Geometry check sheet. Reference: the model listing, model coordinates, mm. Face numbers are marked on the shaded views. A direction names the side the tool comes from. Give positions to 0.01 mm unless a question says otherwise; leave off trailing zeros. Write each loop counter-clockwise with the first axis right and the second up, starting at its lowest first coordinate (ties: lowest second). Pieces come first, ordered by that corner, then holes. Notation, with made-up numbers: (62, -14.5) -> (105, -14.5) arc R16 ccw to (105, -8.5) -> close; hole circle Ø11 at (47.25, -4.75). An arc over 180 degrees is marked (long way). Write item = value, one per line. Start each with the question number.
1. Mould release check, pull along X, two halves, no side actions. Record for the marked faces 1, 2, 3 and 4: pulls with the +X half, pulls with the -X half, needs draft (parallel to the pull), parting line crosses it, or undercut.
2. Depth check by flat-ended pin: P1, Ø2.5, axis at x = 3.5, y = 17.5, coming from the -Z side; P2, Ø1.4, axis at x = -10, z = -10.5, coming from the -Y side; P3, Ø1.6, axis at y = 17, z = 4, coming from the -X side. Enter the tip coordinate at first touch or a pass-through.
3. Cross-section at D-D, the plane y = 17. Record the cut outline in (x, z), plus the area to 3 significant figures.
4. Thickness scan on line 1 along Z through (x, y) = (10.25, 8); line 2 along Z through (x, y) = (-10.75, 6.25); line 3 along X through (y, z) = (9.25, -9.75). Record the ranges inside material, lowest first.
5. Set-up check for the marked faces 5 and 6: record each of +Z, -Z, +X, -X, +Y, -Y from which the full face is reachable in a straight line by a thin tool's end or side.
6. Cross-section at A-A, the plane y = 3.5. Record the cut outline in (x, z).
```python
from build123d import *

# Parameters (mm, degrees)
F0_W     = 25.4
F0_H     = 25.4
F1_DEPTH = 19.05
F2_R     = 7.9375
F3_DEPTH = 25.401
F4_W     = 25.4
F4_H     = 25.4
F4_W_2   = 22.225
F4_H_2   = 22.225
F5_DEPTH = 3.175
F6_R     = 1.35255
F7_DEPTH = 12.7


with BuildPart() as f1:
    # F0 (on Front) → F1 (new body)
    with BuildSketch(Plane.XZ):
        Rectangle(F0_W, F0_H)
    extrude(amount=-F1_DEPTH)

    # F2 (on face) → F3 (cut, through all)
    with BuildSketch(Plane.XY.offset(12.7)):
        Circle(F2_R)
    extrude(amount=-F3_DEPTH, mode=Mode.SUBTRACT)

    # F4 (on face) → F5 (cut)
    with BuildSketch(Plane(origin=(0, 19.05, 0), x_dir=(-1, 0, 0), z_dir=(0, 1, 0))):
        Rectangle(F4_W, F4_H)
        Rectangle(F4_W_2, F4_H_2, mode=Mode.SUBTRACT)
    extrude(amount=-F5_DEPTH, mode=Mode.SUBTRACT)

    # F6 (on face) → F7 (cut)
    with BuildSketch(Plane.XZ):
        with Locations((-10.31748, 10.31748)):
            Circle(F6_R)
        with Locations((-10.31748, -10.31748)):
            Circle(F6_R)
        with Locations((10.31748, 10.31748)):
            Circle(F6_R)
        with Locations((10.31748, -10.31748)):
            Circle(F6_R)
    extrude(amount=-F7_DEPTH, mode=Mode.SUBTRACT)


solid = f1.part
```
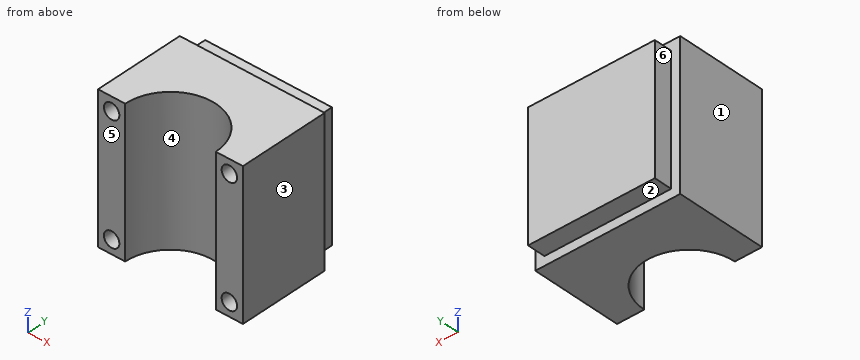
Answers:
q1.face_1 = pulls with the -X half
q1.face_2 = needs draft
q1.face_3 = pulls with the +X half
q1.face_4 = undercut
q2.P1 = -11.11
q2.P2 = 12.7
q2.P3 = -11.11
q3.outline = (-11.11, -11.11) -> (11.11, -11.11) -> (11.11, 11.11) -> (-11.11, 11.11) -> close
q3.area = 494 mm^2
q4.line_1 = -12.7 to -11.67, -8.97 to 8.97, 11.67 to 12.7
q4.line_2 = -12.7 to -11.6, -9.04 to 9.04, 11.6 to 12.7
q4.line_3 = -12.7 to -11.55, -9.09 to 9.09, 11.55 to 12.7
q5.face_5 = +Z, -Z, +X, -X, -Y
q5.face_6 = +Z, -Z, -X, +Y
q6.outline = (-12.7, -12.7) -> (-7.12, -12.7) -> (-7.12, 12.7) -> (-12.7, 12.7) -> close; (7.12, -12.7) -> (12.7, -12.7) -> (12.7, 12.7) -> (7.12, 12.7) -> close; hole circle Ø2.71 at (-10.32, -10.32); hole circle Ø2.71 at (-10.32, 10.32); hole circle Ø2.71 at (10.32, -10.32); hole circle Ø2.71 at (10.32, 10.32)
